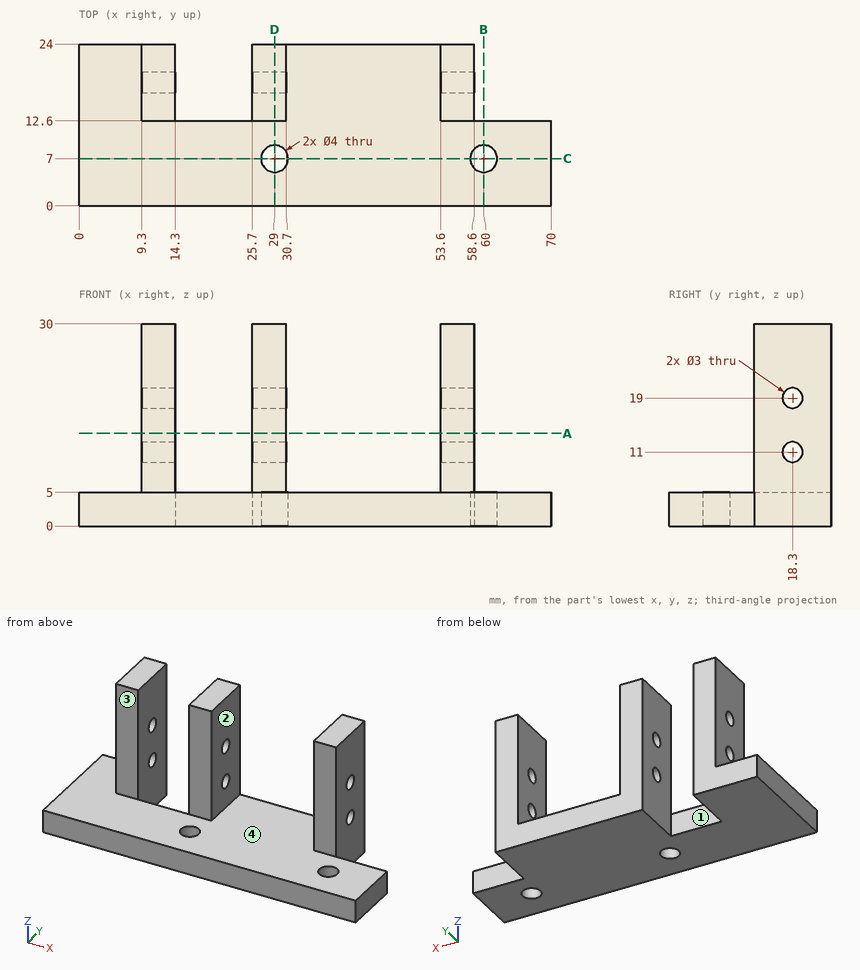
Drawing for the job (mm, zero at the part's lowest x, y, z). A direction names the side the tool comes from. Coordinates: 2 decimals unless noted, no trailing zeros. Write each loop counter-clockwise with the first axis right and the second up, starting at its lowest first coordinate (ties: lowest second). Pieces come first, ordered by that corner, then holes. Notation, with made-up numbers: (46, 19.5) - (73, 19.5) arc R36 ccw to (73, 54.5) - close; hole circle Ø5 at (-17.5, 33). An arc over 180 degrees is marked (long way). Write each question's results on one line, items separated by ' | '. Start each with the question number.
1) Cut at A-A (z = 13.75). Write the cut outline in (x, y), then the cut area to 3 significant figures.
2) Cut at D-D (x = 29). Write the cut outline in (y, z).
3) Cut at B-B (x = 60). Write the cut outline in (y, z).
4) Flat gauge pins, fed straight in: P1, Ø3, axis at x = 50.5, z = 21.5, coming from the +Y side; P2, Ø12.5, axis at y = 18.5, z = 8, coming from the +X side; P3, Ø6.5, axis at x = 29, y = 7, coming from the +Z side; P4, Ø3, axis at y = 13, z = 10.5, coming from the -X side. Where does each tip first touch, or does it go through?
5) Probe line 1 along X through (y, z) = (20, 22.5); line 2 along Z through (x, y) = (54.7, 18.3); line 3 along Z through (x, y) = (32, 17). List the from-to ranges inside material, lowest first. Write a range as from..to.
6) Cut at C-C (y = 7). Write the cut outline in (x, z).
7) 3-axis set-ups, long thin cutter, end or side, ignore diameter. For the marked faces 1, 2, 3 and 4: which of +Z, -Z, +X, -X, +Y, -Y reach the whole face in a straight line?
Returned:
1) outline: (9.3, 12.6) - (14.3, 12.6) - (14.3, 24) - (9.3, 24) - close; (25.7, 12.6) - (30.7, 12.6) - (30.7, 24) - (25.7, 24) - close; (53.6, 12.6) - (58.6, 12.6) - (58.6, 24) - (53.6, 24) - close | area: 171 mm^2
2) outline: (0, 0) - (5, 0) - (5, 5) - (0, 5) - close; (9, 0) - (24, 0) - (24, 30) - (12.6, 30) - (12.6, 5) - (9, 5) - close; hole circle Ø3 at (18.3, 11); hole circle Ø3 at (18.3, 19)
3) outline: (0, 0) - (5, 0) - (5, 5) - (0, 5) - close; (9, 0) - (12.6, 0) - (12.6, 5) - (9, 5) - close
4) P1: through | P2: x = 58.6 | P3: z = 5 | P4: x = 9.3
5) line 1: 9.3..14.3, 25.7..30.7, 53.6..58.6 | line 2: 0..9.5, 12.5..17.5, 20.5..30 | line 3: 0..5
6) outline: (0, 0) - (27, 0) - (27, 5) - (0, 5) - close; (31, 0) - (58, 0) - (58, 5) - (31, 5) - close; (62, 0) - (70, 0) - (70, 5) - (62, 5) - close
7) face 1: +Z, -Z, +Y | face 2: +Z, +Y, -Y | face 3: +Z, +X, -X, -Y | face 4: +Z, -Y
